Read the model definition and answer for the solid it produces. Units are mm, in the model's axes. A direction names the side the tool comes from. Give positions to 0.01 mm unless a question says otherwise; leave off trailing zeros. Loops run counter-clockwise (first coordinate to the right, second up) from the corner with the lowest first, then second, coordinate; pieces in that order, holes last. Notation, with made-up numbers: (70.5, 30) -> (100.5, 30) arc R10 cw to (100.5, 38) -> close; hole circle Ø5 at (48.5, 8.5). An arc over 180 degrees is marked (long way). Answer as CSV lines item,"result". Start each with the question number.
```python
from build123d import *

# Parameters (mm, degrees)
CUT_EXTRUDE_1_DEPTH      = 38.436613095
CUT_EXTRUDE_1_DEPTH_BACK = 38.436613095
SKETCH_2_R               = 12.5
FILLET_1_R               = 1
FILLET_2_R               = 0.5
FILLET_3_R               = 1


with BuildPart() as part:
    # Эскиз1 → Повернуть1 (revolve)
    with BuildSketch(Plane.XY, mode=Mode.PRIVATE) as revolve_1_sk:
        Polygon((-4, 33), (-4, 16), (-7, 16), (-7, -7), (-10, -7), (-10, 23), (-12.5, 23), (-12.5, 33), align=None)
    revolve(revolve_1_sk.sketch.rotate(Axis((0, 98.834265919, 0), (0, -1, 0)), 270), axis=Axis((0, 98.834265919, 0), (0, -1, 0)))

    # Эскиз2 → Вырез-Вытянуть1 (cut, two sides: drawn at the far end of the back side and taken through both)
    with BuildSketch(Plane.XY.offset(-CUT_EXTRUDE_1_DEPTH_BACK)):
        with Locations((0, 40.5)):
            Circle(SKETCH_2_R)
    extrude(amount=CUT_EXTRUDE_1_DEPTH + CUT_EXTRUDE_1_DEPTH_BACK, mode=Mode.SUBTRACT)

    # Скругление1
    fillet_1_edges = [part.edges().sort_by_distance(p)[0] for p in [
        (12.5, 33, 0),
        (-12.5, 33, 0),
    ]]
    fillet(fillet_1_edges, radius=FILLET_1_R)

    # Скругление2
    fillet_2_edges = [part.edges().sort_by_distance(p)[0] for p in [
        (0, 23, -12.5),
    ]]
    fillet(fillet_2_edges, radius=FILLET_2_R)

    # Скругление3
    fillet_3_edges = [part.edges().sort_by_distance(p)[0] for p in [
        (0, -7, -10),
        (0, -7, -7),
    ]]
    fillet(fillet_3_edges, radius=FILLET_3_R)


solid = part.part
```
(1) A tool of negligible diameter and unlimited length cuts with its end or side. For faces 1 (the face through (9.76, 8.7, -2.17)), 2 (the face through (-11, 33, 0)), from which of +Z, -Z, +X, -X, +Y, -Y can it reach the whole face along a straight path? Write none if from no direction.
(2) Find section A-A on x = 0. Write down the section's boundary in (y, z), then the cut area to 3 significant figures.
(3) Find section D-D on y = 30. Write down the section's boundary in (x, z).
(4) The mould has two halves that part along Z. Classify faces 3 (the face through (6.834, 4.846, -1.517)), 4 (the face through (-8.45, 26.87, -9.21)), 5 (the face through (-9, 23, 5)): pulls with the +Z half, pulls with the -Z half, needs draft (parallel to the pull), parting line crosses it, or undercut.
(5) Find section C-C on y = 2.5. Write down the section's boundary in (x, z).
(6) Find the intervals of material crossed by line 1 along X through (y, z) = (22.5, -0.25); line 2 along X through (y, z) = (9, 0); line 3 along Y through (x, z) = (0, -8.25), in increasing order. Write a range as from..to.
(7) Each of these flat-tipped pins is pushed along its axis until it touches: P1, Ø4, axis at x = 3, z = 1, coming from the -Y side; P2, Ø10, axis at y = 6, z = -4.5, coming from the -X side; P3, Ø4, axis at x = -1, y = 20.5, coming from the -Z side. Where does it stop, or does it pass through?
(8) Find section B-B on z = 0. Write down the section's boundary in (x, y), then the cut area to 3 significant figures.
Answer block:
1,face 1,"-Y"
1,face 2,"+Z, -Z, +X, -X, +Y"
2,outline,"(-7, -9) arc R1 ccw to (-6, -10) -> (23, -10) -> (23, -12) arc R0.5 ccw to (23.5, -12.5) -> (28, -12.5) -> (28, -4) -> (16, -4) -> (16, -7) -> (-6, -7) arc R1 ccw to (-7, -8) -> close; (-7, 8) arc R1 ccw to (-6, 7) -> (16, 7) -> (16, 4) -> (28, 4) -> (28, 12.5) -> (23.5, 12.5) arc R0.5 ccw to (23, 12) -> (23, 10) -> (-6, 10) arc R1 ccw to (-7, 9) -> close"
2,area,"306 mm2"
3,outline,"(-6.78, -10.5) -> (-6.78, 10.5) arc R12.5 ccw to start; (6.78, -10.5) arc R12.5 ccw to (6.78, 10.5) -> close"
4,face 3,"undercut"
4,face 4,"parting line crosses it"
4,face 5,"needs draft"
5,outline,"circle Ø20 at (0, 0); hole circle Ø14 at (0, 0)"
6,line 1,"x = -10..-3.99, 3.99..10"
6,line 2,"x = -10..-7, 7..10"
6,line 3,"y = -7..28"
7,P1,"stops at y = 16"
7,P2,"stops at x = -10"
7,P3,"stops at z = -10"
8,outline,"(-12.5, 23.5) arc R0.5 ccw to (-12, 23) -> (-10, 23) -> (-10, -6) arc R1 ccw to (-9, -7) -> (-8, -7) arc R1 ccw to (-7, -6) -> (-7, 16) -> (-4, 16) -> (-4, 28.66) arc R12.5 cw to (-10, 33) -> (-11.5, 33) arc R1 ccw to (-12.5, 32) -> close; (4, 16) -> (7, 16) -> (7, -6) arc R1 ccw to (8, -7) -> (9, -7) arc R1 ccw to (10, -6) -> (10, 23) -> (12, 23) arc R0.5 ccw to (12.5, 23.5) -> (12.5, 32) arc R1 ccw to (11.5, 33) -> (10, 33) arc R12.5 cw to (4, 28.66) -> close"
8,area,"359 mm2"
